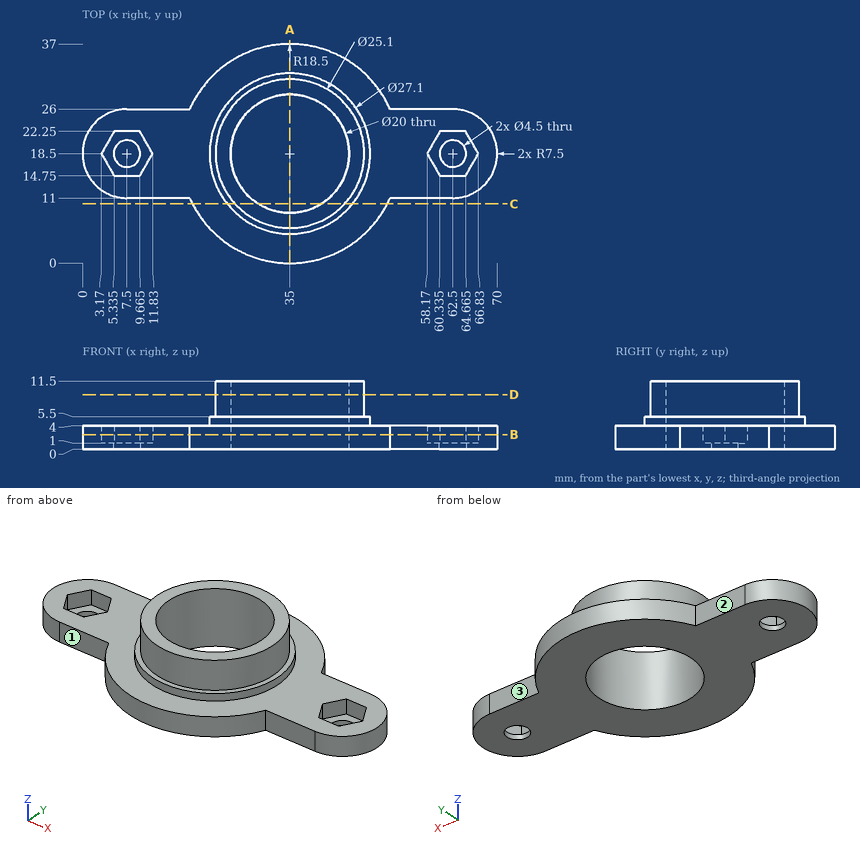
The figure shows three views and two pictorial views of one solid part (mm, origin at its lowest corner). Answer the questions. A direction names the side the tool comes from. Round coordinates to 2 decimals unless told otherwise and drop trailing zeros. Write each loop counter-clockwise with the first axis right and the second up, starting at its lowest first coordinate (ties: lowest second). Pieces come first, ordered by that corner, then holes. Notation, with made-up numbers: (39.5, 63.25) - (65.5, 63.25) arc R14 cw to (65.5, 86.25) - close; hole circle Ø2 at (-24, 80.5). An arc over 180 degrees is marked (long way). Answer in a Markdown table with one row per item. Add a question column.
1. A cutting plane is placed at B-B, the plane z = 2.5. Count the separate pieces of the cut face and the enclosed holes in it, and give its area (3 significant figures).
2. Given pin 1 (4 mm diameter, centred on x = 7.5, y = 18.5, fed in from -Z); pin 2 (1.5 mm diameter, centred on x = 62, z = 2, fed in from +Y); pin 3 (6 mm diameter, centred on y = 32, z = 8.5, fed in from -X); pin 4 (5 mm diameter, centred on x = 62.5, y = 18.5, fed in from -Z), each flat-ended and moving along its own axis, determine where each tip first touches the part or whether it passes through.
3. A cutting plane is placed at D-D, the plane z = 9.25. Determine the outline of the cut face in (x, y).
4. A cutting plane is placed at A-A, the plane x = 35. Determine the outline of the cut face in (y, z), and give its area (3 significant figures).
5. A cutting plane is placed at C-C, the plane y = 10. Determine the outline of the cut face in (x, z), and give its area (3 significant figures).
6. For the marked faces 1, 2 and 3, determine the directions among +Z, -Z, +X, -X, +Y, -Y from which every point of the face is accessible in a straight line to the end or side of a thin tool.
7. Find the intervals of material crossed by line 1 along Y through (x, z) = (7.5, 0.6); line 2 along X through (y, z) = (20, 2.5); line 3 along Z through (x, y) = (49.5, 23), in increasing order. Write a range as from..to.
Worked out:
| question | item | result |
|---|---|---|
| 1 | separate pieces | 1 |
| 1 | enclosed holes | 3 |
| 1 | area | 1,130 mm^2 |
| 2 | pin 1 | through |
| 2 | pin 2 | y = 26 |
| 2 | pin 3 | x = 28.13 |
| 2 | pin 4 | z = 0 |
| 3 | outline | circle Ø25.1 at (35, 18.5); hole circle Ø20 at (35, 18.5) |
| 4 | outline | (0, 0) - (8.5, 0) - (8.5, 11.5) - (5.95, 11.5) - (5.95, 5.5) - (4.95, 5.5) - (4.95, 4) - (0, 4) - close; (28.5, 0) - (37, 0) - (37, 4) - (32.05, 4) - (32.05, 5.5) - (31.05, 5.5) - (31.05, 11.5) - (28.5, 11.5) - close |
| 4 | area | 109 mm^2 |
| 5 | outline | (18.57, 0) - (29.73, 0) - (29.73, 11.5) - (25.77, 11.5) - (25.77, 5.5) - (24.45, 5.5) - (24.45, 4) - (18.57, 4) - close; (40.27, 0) - (51.43, 0) - (51.43, 4) - (45.55, 4) - (45.55, 5.5) - (44.23, 5.5) - (44.23, 11.5) - (40.27, 11.5) - close |
| 5 | area | 153 mm^2 |
| 6 | face 1 | +Z, -Z, -X, -Y |
| 6 | face 2 | +Z, -Z, -X, +Y |
| 6 | face 3 | +Z, -Z, +X, +Y |
| 7 | line 1 | 11..16.25, 20.75..26 |
| 7 | line 2 | 0.15..4.04, 10.96..25.11, 44.89..59.04, 65.96..69.85 |
| 7 | line 3 | 0..4 |
